Work out the finished part from the listing and answer in its coordinate system (mm). A direction names the side the tool comes from. Give positions to 0.01 mm unless a question says otherwise; leave off trailing zeros. Loops run counter-clockwise (first coordinate to the right, second up) from the corner with the lowest first, then second, coordinate; pieces in that order, holes last. Notation, with made-up numbers: (33, 81) - (37, 81) arc R34 cw to (37, 112) - close; hole circle Ø7 at (46.25, 21). An arc over 180 degrees is marked (long way). One line per question, with ' | ' between items.
from build123d import *

# Parameters (mm, degrees)
F0_W     = 35
F0_H     = 15.5
F1_DEPTH = 3
F2_R     = 1.25
F3_DEPTH = 12.5
F5_DEPTH = 2


# Not quite as in the source:
# - a feature names something its author has since deleted; it is built from what else it names


with BuildPart() as f1:
    # F0 (on Top) → F1 (new body, symmetric)
    with BuildSketch(Plane.XY):
        Polygon((-49, 0), (-57, 0), (-57, -2), (-1.0886418074, -2), (-1.0886418074, 0), (-10, 0), (-10, 17.5), (-49, 17.5), align=None)
        with Locations((-29.5, 7.75)):
            Rectangle(F0_W, F0_H, mode=Mode.SUBTRACT)
    extrude(amount=F1_DEPTH, both=True)

    # F2 (on face) → F3 (cut, symmetric)
    with BuildSketch(Plane.XZ.offset(2)):
        with Locations((-54.0886418074, 0)):
            Circle(F2_R)
        with Locations((-5.0886418074, 0)):
            Circle(F2_R)
    extrude(amount=F3_DEPTH, both=True, mode=Mode.SUBTRACT)

    # F4 (on Front) → F5 (join)
    with BuildSketch(Plane.XZ):
        Polygon((-13.2752051018, -17.5318677962), (-13.2752051018, -2.6883990917), (-18.2752051018, -2.6883990917), (-18.2752051018, -3.858309805), (-18.2752051018, -17.5318677962), align=None)
    extrude(amount=F5_DEPTH)


solid = f1.part
1. Find section D-D on y = -1. Write down the section's boundary in (x, z), then the cut area to 3 significant figures.
Evaluation:
outline: (-57, -3) - (-18.28, -3) - (-18.28, -17.53) - (-13.28, -17.53) - (-13.28, -3) - (-1.09, -3) - (-1.09, 3) - (-57, 3) - close; hole circle Ø2.5 at (-54.09, 0); hole circle Ø2.5 at (-5.09, 0) | area: 398 mm2
2. Find section A-A on z = 0. Write down the section's boundary in (x, y), then the cut area to 3 significant figures.
Evaluation:
outline: (-57, -2) - (-55.34, -2) - (-55.34, 0) - (-57, 0) - close; (-52.84, -2) - (-6.34, -2) - (-6.34, 0) - (-10, 0) - (-10, 17.5) - (-49, 17.5) - (-49, 0) - (-52.84, 0) - close; (-3.84, -2) - (-1.09, -2) - (-1.09, 0) - (-3.84, 0) - close; hole (-47, 0) - (-12, 0) - (-12, 15.5) - (-47, 15.5) - close | area: 242 mm2
3. Flat-ended cylindrical pins translate along their axes: pin 1 (3 mm diameter, centred on x = -5.09, z = 0, fed in from +Y); pin 2 (2 mm diameter, centred on x = -54.09, z = 0, fed in from +Y); pin 3 (1.6 mm diameter, centred on y = -1, z = -7.5, fed in from +X); pin 4 (10 mm diameter, centred on x = -16, y = 7.5, fed in from -Z). Find the tip coordinate at first contact, or state that the pin passes through.
Evaluation:
pin 1: y = 0 | pin 2: through | pin 3: x = -13.28 | pin 4: z = -3
4. Which of the six approach directions +Z, -Z, +X, -X, +Y, -Y give full straight-line access (tool end or side, diameter ignored) to faces 5 (the flat face through (-25.9, 0, -2.6)), 6 (the flat face through (-6.5, 0, 0)), 7 (the flat face through (-18.275, -1, -10)), 8 (the flat face through (-53, 0, 1)), 9 (the flat face through (-13.275, -1, -10))?
Evaluation:
face 5: +Z, -Z | face 6: +Z, -Z, +X, +Y | face 7: -Z, -X, +Y, -Y | face 8: +Z, -Z, -X, +Y | face 9: -Z, +X, +Y, -Y
5. Find section B-B on y = 4.5. Write down the section's boundary in (x, z), then the cut area to 3 significant figures.
Evaluation:
outline: (-49, -3) - (-47, -3) - (-47, 3) - (-49, 3) - close; (-12, -3) - (-10, -3) - (-10, 3) - (-12, 3) - close | area: 24.0 mm2
6. Find section C-C on x = -22.5. Write down the section's boundary in (y, z), then the cut area to 3 significant figures.
Evaluation:
outline: (-2, -3) - (0, -3) - (0, 3) - (-2, 3) - close; (15.5, -3) - (17.5, -3) - (17.5, 3) - (15.5, 3) - close | area: 24.0 mm2
7. Determine the mould class of faces 1 (the flat face through (-47, 8, 0)), 2 (the flat face through (-30, 15.5, 0)), 3 (the flat face through (-57, -1, 0)), 4 (the flat face through (-29, 17.5, 0)) for opening direction X: +X half, -X half, draft (parallel to the pull), parting line (faces both ways), or undercut.
Evaluation:
face 1: undercut | face 2: undercut | face 3: -X half | face 4: draft
8. Consider L1, parallel to X at y = 15.25, z = 0; L2, parallel to Z at x = -35.5, y = -0.25; L3, parallel to Y at x = -50, z = -2. Determine where each line is inside the solid, lowest interval first.
Evaluation:
L1: -49 to -47, -12 to -10 | L2: -3 to 3 | L3: -2 to 0
